Check sheet for the modelled part. Datum: model origin and axes. Units: mm. Coordinates: 2 decimals unless noted, no trailing zeros. Write each loop counter-clockwise with the first axis right and the second up, starting at its lowest first coordinate (ties: lowest second). Pieces come first, ordered by that corner, then holes. Notation, with made-up numbers: (33.5, 87.25) -> (42.5, 87.25) arc R33 cw to (42.5, 117.25) -> close; hole circle Ø7 at (89, -33.75). An arc over 180 degrees is marked (long way). One line per item, written item: value. Start each with the question number.
1) Draft check along Z on faces 1 (the flat face through (-19.807, -3.944, 38.241)), 2 (the cylindrical face through (-10.404, -3.944, 70.074)), 3 (the flat face through (65, -4, 52)). Enter one of: +Z half, -Z half, draft (parallel to the pull), parting line (faces both ways), or undercut.
2) Sectioned sample at A-A on x = 20. Enter the section's corners in (y, z).
3) Sectioned sample at D-D on z = 67. Enter the section's corners in (x, y).
4) Sectioned sample at B-B on z = -20. Enter the section's corners in (x, y), plus the area to 3 significant figures.
5) Sectioned sample at C-C on y = -5.75. Give the number of separate pieces and of enclosed holes in the cut face, plus the area to 3 significant figures.
6) Scan lines: line 1 along Z through (x, y) = (0, -4.75); line 2 along Z through (x, y) = (60, -1.5); line 3 along Z through (x, y) = (-10, -2.5). Record each from-to range of solid material in increasing order. Write a range as [from, to].
7) Gauge pin test, flat ends, axial feed: P1, Ø2, axis at y = -6, z = 6.5, coming from the +X side; P2, Ø3, axis at y = -5.5, z = 3, coming from the +X side; P3, Ø4, axis at y = -1, z = 50.5, coming from the -X side. Record the tip position at first contact, or that the pin passes through.
```python
from build123d import *

# Parameters (mm, degrees)
F0_R     = 2.25
F0_R_2   = 8.05
F0_R_3   = 3.1
F1_DEPTH = 8


with BuildPart() as f1:
    # F0 (on Front) → F1 (new body)
    with BuildSketch(Plane.XZ):
        with BuildLine():
            Line((65, 72), (-15, 72))
            Line((-15, 72), (-24.750349, 3.524233))
            ThreePointArc((-24.750349, 3.524233), (-10.901742, -22.497822), (18.103448, -17.241379))
            Line((18.103448, -17.241379), (65, 32))
            Line((65, 32), (65, 72))
        make_face()
        with Locations((0, -20)):
            Circle(F0_R, mode=Mode.SUBTRACT)
        with Locations((-20, 0)):
            Circle(F0_R, mode=Mode.SUBTRACT)
        Circle(F0_R_2, mode=Mode.SUBTRACT)
        with Locations((0, 20)):
            Circle(F0_R, mode=Mode.SUBTRACT)
        with Locations((20, 0)):
            Circle(F0_R, mode=Mode.SUBTRACT)
        with Locations((-10, 37)):
            Circle(F0_R_3, mode=Mode.SUBTRACT)
        with Locations((-10, 67)):
            Circle(F0_R_3, mode=Mode.SUBTRACT)
        with Locations((60, 37)):
            Circle(F0_R_3, mode=Mode.SUBTRACT)
        with Locations((60, 67)):
            Circle(F0_R_3, mode=Mode.SUBTRACT)
    extrude(amount=F1_DEPTH)


solid = f1.part
```
Answers:
1. face 1: +Z half
1. face 2: undercut
1. face 3: draft
2. outline: (-8, -15.25) -> (0, -15.25) -> (0, -2.25) -> (-8, -2.25) -> close; (-8, 2.25) -> (0, 2.25) -> (0, 72) -> (-8, 72) -> close
3. outline: (-15.71, -8) -> (-13.1, -8) -> (-13.1, 0) -> (-15.71, 0) -> close; (-6.9, -8) -> (56.9, -8) -> (56.9, 0) -> (-6.9, 0) -> close; (63.1, -8) -> (65, -8) -> (65, 0) -> (63.1, 0) -> close
4. outline: (-15, -8) -> (-2.25, -8) -> (-2.25, 0) -> (-15, 0) -> close; (2.25, -8) -> (15, -8) -> (15, 0) -> (2.25, 0) -> close
4. area: 204 mm2
5. separate pieces: 1
5. enclosed holes: 9
5. area: 6,290 mm2
6. line 1: z = [-25, -22.25], [-17.75, -8.05], [8.05, 17.75], [22.25, 72]
6. line 2: z = [26.75, 33.9], [40.1, 63.9], [70.1, 72]
6. line 3: z = [-22.91, 33.9], [40.1, 63.9], [70.1, 72]
7. P1: stops at x = 41.67
7. P2: stops at x = 38.81
7. P3: stops at x = -18.35
